Here's the drawing with two shaded views (mm, measured from the low corner). I have some questions. A direction names the side the tool comes from. Round coordinates to 2 decimals unless told otherwise and drop trailing zeros. Loops run counter-clockwise (first coordinate to the right, second up) from the corner with the lowest first, then second, coordinate; pieces in that order, holes last. Notation, with made-up numbers: M 37,25 L 53,25 A11 ccw 53,39 Z; hole C -30.75,36 d3. An arc over 180 degrees is marked long. One line per item, written item: value. Start each with the question number.
Q1. Thinking about a two-plate mould opening in X: for the marked faces 3, 4 and 5, which applies, released by +X, released by -X, zero draft, split by the parting line, or undercut?
Q2. Imagine slicing it at C-C (x = 8). Please give me the cut outline in (y, z), then the cut area to 3 significant figures.
Q3. I'm going to push flat-ended pins straight in: pin 1 Ø8.5 at (x, y) = (15.875, 19.05) entering from +Z; pin 2 Ø11 at (x, z) = (26.67, 11.43) entering from +Y. Where does each tip first touch, or does it pass through?
Q4. Please list where these lines run through material, in increasing order: line 1 along X through (y, z) = (2.75, 7.62); line 2 along Z through (x, y) = (5, 3.5); line 3 along X through (y, z) = (1.45, 11.43).
Q5. Imagine slicing it at B-B (z = 7.62). Please give me the cut outline in (x, y).
Q6. Imagine slicing it at D-D (y = 3). Please give me the cut outline in (x, z).
Q7. Which directions (+Z, -Z, +X, -X, +Y, -Y) give clear straight access to the entire face, cutting with the end or side of a thin tool? Please do the marked faces 1 and 2.
Q8. Imagine slicing it at A-A (y = 19.05). Please give me the cut outline in (x, z).
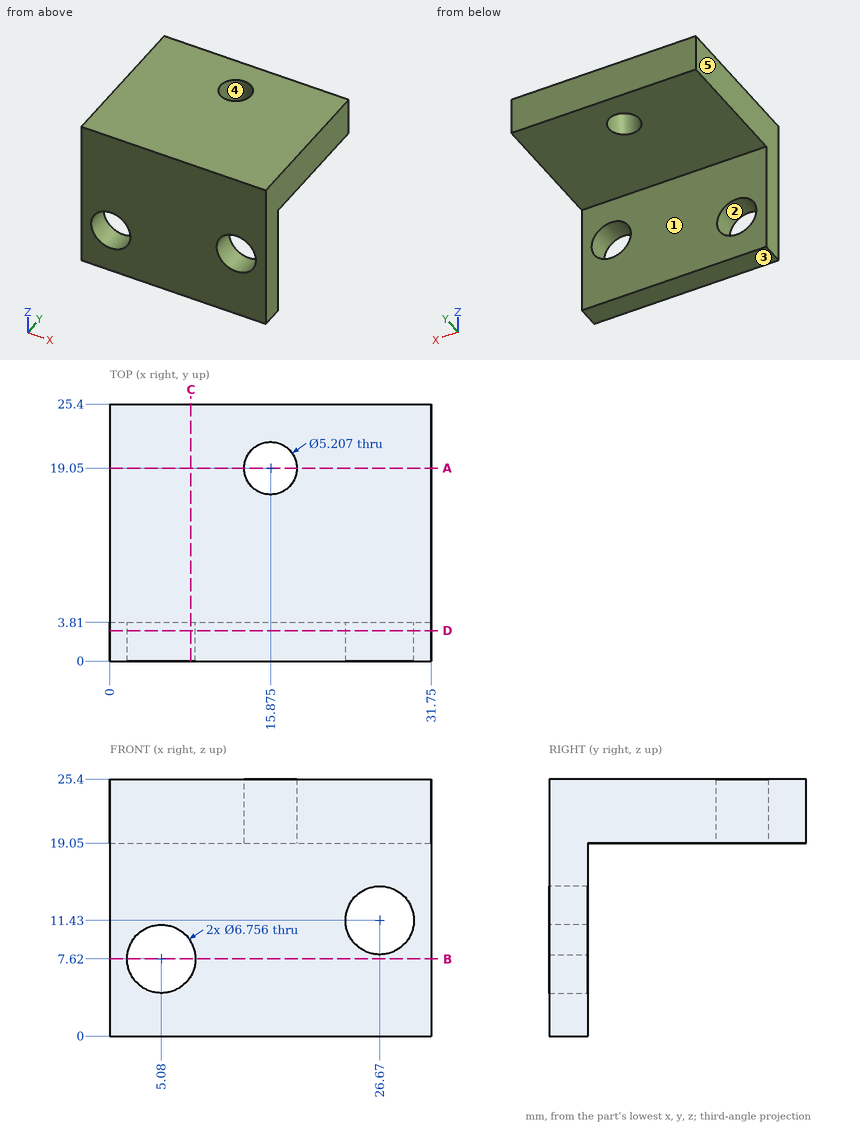
Report:
1. face 3: zero draft
1. face 4: undercut
1. face 5: released by -X
2. outline: M 0,0 L 3.81,0 L 3.81,5.92 L 0,5.92 Z; M 0,9.32 L 3.81,9.32 L 3.81,19.05 L 25.4,19.05 L 25.4,25.4 L 0,25.4 Z
2. area: 221 mm²
3. pin 1: stops at z = 25.4
3. pin 2: stops at y = 3.81
4. line 1: x = 0 to 1.7, 8.46 to 31.75
4. line 2: z = 0 to 4.24, 11 to 25.4
4. line 3: x = 0 to 23.29, 30.05 to 31.75
5. outline: M 0,0 L 1.7,0 L 1.7,3.81 L 0,3.81 Z; M 8.46,0 L 31.75,0 L 31.75,3.81 L 8.46,3.81 Z
6. outline: M 0,0 L 31.75,0 L 31.75,25.4 L 0,25.4 Z; hole C 5.08,7.62 d6.76; hole C 26.67,11.43 d6.76
7. face 1: -Z, +X, -X, +Y
7. face 2: +Y, -Y
8. outline: M 0,19.05 L 13.27,19.05 L 13.27,25.4 L 0,25.4 Z; M 18.48,19.05 L 31.75,19.05 L 31.75,25.4 L 18.48,25.4 Z
